Part model, mm, in its own coordinate system. A direction names the side the tool comes from. Give positions to 0.01 mm unless a question says otherwise; leave off trailing zeros. Order: outer loops, then holes, each group sorted by start corner. A loop starts at its lowest first (then second) coordinate and runs counter-clockwise, first axis right, second up. Notation, with made-up numbers: (55.5, 7) - (111.5, 7) arc R29 cw to (111.5, 27) - close; hole circle Ø5 at (85, 29). An arc over 180 degrees is marked (long way). Use one line per item in the form item = value. Start each with the question number.
1. Pin check, flat tips, straight feed: P1, Ø3, axis at x = 40, y = 26.5, coming from the +Z side; P2, Ø24.5, axis at y = 33.2, z = 0, coming from the -X side; P3, Ø3, axis at x = 27.5, z = -9.5, coming from the +Y side. Stop position of each tip, or through.
2. Drill centre lines: line 1 (Y direction, x = 34.5, z = 0); line 2 (Y direction, x = 21, z = 0); line 3 (Z direction, x = 35, y = 34) (3 decimals). Where is each one in solid material? Low to high.
3. Tool access for faces 1 (the face through (0, 9, -12)), 2 (the face through (43.33, 36, 8)), 3 (the face through (10.414, 33, 0)), 4 (the face through (43.584, 36, -8)): list every direction of +Z, -Z, +X, -X, +Y, -Y with a clear straight run to the whole face (end or side of a thin tool).
4. Band-saw the part on A-A, the plane y = 43. State how many separate pieces and enclosed holes the cut face has, plus the area to 3 significant figures.
5. Pull direction X, two halves, no side cores. Call faces 5 (the face through (38.764, 40.872, -1.704)), 6 (the face through (27.592, 50.647, -22.757)), 7 (the face through (21.38, 62.25, 15.11)): +X half, -X half, draft (parallel to the pull), parting line (faces both ways), or undercut.
6. Band-saw the part on B-B, the plane x = 8.5. List the corners of the cut face in (y, z), plus the area to 3 significant figures.
from build123d import *


with BuildPart() as part:
    # Sketch1 → Revolve14 (revolve)
    with BuildSketch(Plane.XY, mode=Mode.PRIVATE) as revolve14_sk:
        with BuildLine():
            ThreePointArc((38.650867659, 13.552705122), (39.703988191, 13.111091095), (40.764660937, 13.534244884))
            ThreePointArc((40.764660937, 13.534244884), (42.547871865, 17.29449042), (43.330039933, 21.381971408))
            Line((43.330039933, 21.381971408), (43.330039933, 25.3365))
            Line((43.330039933, 25.3365), (43.17780534, 25.3365))
            Line((43.17780534, 25.3365), (43.097253999, 25.231839758))
            ThreePointArc((43.097253999, 25.231839758), (29.037172994, 13.950323802), (11.365936374, 10.3886))
            Line((11.365936374, 10.3886), (11.365936374, 4.5212))
            Line((11.365936374, 4.5212), (43.369936374, 4.5212))
            Line((43.369936374, 4.5212), (43.369936374, 0))
            Line((43.369936374, 0), (0, 0.889))
            Line((0, 0.889), (0, 6.477))
            Line((0, 6.477), (10.414, 10.3886))
            Line((10.414, 10.3886), (10.414, 33.1978))
            Line((10.414, 33.1978), (10.718952979, 33.1978))
            Line((10.718952979, 33.1978), (10.718952979, 10.6426))
            Line((10.718952979, 10.6426), (11.370994965, 10.6426))
            ThreePointArc((11.370994965, 10.6426), (28.898518318, 14.165897296), (42.857219331, 25.3365))
            Line((42.857219331, 25.3365), (34.784736374, 25.3365))
            Line((34.784736374, 25.3365), (34.784736374, 25.5905))
            Line((34.784736374, 25.5905), (46.341736374, 25.5905))
            Line((46.341736374, 25.5905), (46.341736374, 25.3365))
            ThreePointArc((46.341736374, 25.3365), (45.079355578, 25.408427544), (43.815899343, 25.358857493))
            ThreePointArc((43.815899343, 25.358857493), (43.650770462, 25.277423096), (43.584039933, 25.105824305))
            Line((43.584039933, 25.105824305), (43.584039933, 21.3741))
            ThreePointArc((43.584039933, 21.3741), (42.78607195, 17.205705338), (40.963051574, 13.3731))
            ThreePointArc((40.963051574, 13.3731), (39.717157055, 12.857033593), (38.471262536, 13.3731))
            Line((38.471262536, 13.3731), (38.650867659, 13.552705122))
        make_face()
    revolve(revolve14_sk.sketch.rotate(Axis((10.414, 33.1978, 0), (1, 0, 0)), 270), axis=Axis((10.414, 33.1978, 0), (1, 0, 0)))


solid = part.part
From the geometry:
q1.P1 = 32.72
q1.P2 = 10.41
q1.P3 = 65.08
q2.line_1 = 0.18 to 4.52, 17.08 to 17.39, 49.01 to 49.32, 61.87 to 66.21
q2.line_2 = 0.46 to 4.52, 11.23 to 11.49, 54.9 to 55.16, 61.87 to 65.94
q2.line_3 = -33.016 to -28.665, -15.748 to -15.435, -7.82 to -7.565, 7.565 to 7.82, 15.435 to 15.748, 28.665 to 33.016
q3.face_1 = +Z, -Z, -X, +Y, -Y
q3.face_2 = none
q3.face_3 = -X
q3.face_4 = +X
q4.separate_pieces = 2
q4.enclosed_holes = 1
q4.area = 520 mm²
q5.face_5 = undercut
q5.face_6 = draft
q5.face_7 = -X half
q6.outline = circle Ø64.97 at (33.2, 0); hole circle Ø47.06 at (33.2, 0)
q6.area = 1,580 mm²
